from build123d import *

# Parameters (mm, degrees)
BOSS_EXTRUDE1_DEPTH                                = 25.4
FILLET1_R                                          = 19.05
CSK_FOR_10_FLAT_HEAD_MACHINE_SCREW_100_D           = 5.1054
CSK_FOR_10_FLAT_HEAD_MACHINE_SCREW_100_CSINK_D     = 9.779
CSK_FOR_10_FLAT_HEAD_MACHINE_SCREW_100_CSINK_ANGLE = 100


with BuildPart() as part:
    # Sketch1 → Boss-Extrude1 (new body)
    with BuildSketch(Plane.XY):
        Polygon((-323.85, 279.4), (323.85, 279.4), (323.85, -76.2), (228.6, -76.2), (228.6, 0), (-228.6, 0), (-228.6, -76.2), (-323.85, -76.2), align=None)
    extrude(amount=BOSS_EXTRUDE1_DEPTH)

    # Fillet1
    fillet1_edges = [part.edges().sort_by_distance(p)[0] for p in [
        (228.6, -76.2, 12.7),
        (228.6, 0, 12.7),
        (-228.6, 0, 12.7),
        (-228.6, -76.2, 12.7),
    ]]
    fillet(fillet1_edges, radius=FILLET1_R)

    # CSK for #10 Flat Head Machine Screw (100)1 (through all)
    with Locations(Plane.XY.offset(25.4)):
        with Locations((0, 266.7), (76.2, 266.7), (152.4, 266.7), (-76.2, 266.7), (-152.4, 266.7)):
            CounterSinkHole(CSK_FOR_10_FLAT_HEAD_MACHINE_SCREW_100_D / 2, CSK_FOR_10_FLAT_HEAD_MACHINE_SCREW_100_CSINK_D / 2, counter_sink_angle=CSK_FOR_10_FLAT_HEAD_MACHINE_SCREW_100_CSINK_ANGLE)


solid = part.part
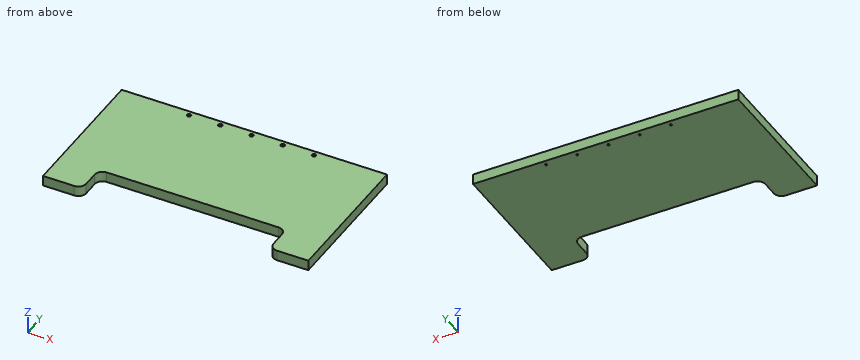
Check sheet for the modelled part. Datum: model origin and axes. Units: mm. Round coordinates to 2 decimals unless told otherwise and drop trailing zeros. Loops run counter-clockwise (first coordinate to the right, second up) from the corner with the lowest first, then second, coordinate; pieces in that order, holes last. Notation, with made-up numbers: (70, 15) -> (99, 15) arc R14 ccw to (99, 22) -> close; hole circle Ø7 at (88, 89.5). An arc over 180 degrees is marked (long way). Put each result on its own line as item: value. Start each with the question number.
1. Scan lines: probe 1 along X at (y, z) = (266.7, 17.5); probe 2 along Y at (x, z) = (76.2, 5.25); probe 3 along X at (y, z) = (-41.5, 11.75). Record each from-to range of solid material in increasing order.
2. Section check A-A (z = 6.25). Enter the section's corners in (x, y).
3. Gauge pin test, flat ends, axial feed: pin 1 (7.5 mm diameter, centred on x = -75, z = 11.5, fed in from -Y); pin 2 (6 mm diameter, centred on x = -76.2, y = 266.7, fed in from +Z); pin 3 (6.5 mm diameter, centred on x = 0, y = 266.7, fed in from +Z). Record the tip position at first contact, or that the pin passes through.
Findings:
1. probe 1: x = -323.85 to -154.95, -149.85 to -78.75, -73.65 to -2.55, 2.55 to 73.65, 78.75 to 149.85, 154.95 to 323.85
1. probe 2: y = 0 to 264.15, 269.25 to 279.4
1. probe 3: x = -323.85 to -228.6, 228.6 to 323.85
2. outline: (-323.85, -76.2) -> (-247.65, -76.2) arc R19.05 ccw to (-228.6, -57.15) -> (-228.6, -19.05) arc R19.05 cw to (-209.55, 0) -> (209.55, 0) arc R19.05 cw to (228.6, -19.05) -> (228.6, -57.15) arc R19.05 ccw to (247.65, -76.2) -> (323.85, -76.2) -> (323.85, 279.4) -> (-323.85, 279.4) -> close; hole circle Ø5.11 at (-152.4, 266.7); hole circle Ø5.11 at (-76.2, 266.7); hole circle Ø5.11 at (0, 266.7); hole circle Ø5.11 at (76.2, 266.7); hole circle Ø5.11 at (152.4, 266.7)
3. pin 1: stops at y = 0
3. pin 2: stops at z = 23.81
3. pin 3: stops at z = 24.02
